Work out the finished part from the listing and answer in its coordinate system (mm). A direction names the side the tool comes from. Coordinates: 2 decimals unless noted, no trailing zeros. Write each loop counter-clockwise with the first axis right and the second up, starting at its lowest first coordinate (ties: lowest second). Pieces come first, ordered by that corner, then holes. Notation, with made-up numbers: (-20, 82) - (2, 82) arc R16 cw to (2, 109) - close; hole circle Ø9 at (37, 62). An arc over 180 degrees is marked (long way). Use one line per item in the form item = value. Start each with the question number.
Item 1: Consider probe 1 along X at (y, z) = (3.25, -6.5); probe 2 along Y at (x, z) = (5.75, -6.25); probe 3 along X at (y, z) = (15.5, -9.25). Determine where each line is inside the solid, lowest interval first.
Item 2: Given pin 1 (2.5 mm diameter, centred on x = 16, z = -8, fed in from +Y); pin 2 (2.5 mm diameter, centred on x = -1.425, z = -7.25, fed in from -Y); pin 3 (5 mm diameter, centred on y = 10.5, z = -1.5, fed in from +X), each flat-ended and moving along its own axis, determine where each tip first touches the part or whether it passes through.
Item 3: A cutting plane is placed at B-B (x = 16.5). Write down the section's boundary in (y, z), then the cut area to 3 significant figures.
Item 4: For faces 5 (the cylindrical face through (8.36, 16.54, -5.02)), 6 (the cylindrical face through (14.398, 7.787, -5.67)), 7 (the flat face through (-3, 0, -7)), 8 (the cylindrical face through (15.31, 1.03, -7.19)), determine the directions among +Z, -Z, +X, -X, +Y, -Y from which every point of the face is accessible in a straight line to the end or side of a thin tool.
Item 5: A cutting plane is placed at D-D (y = 3.5). Write down the section's boundary in (x, z) (3 decimals), then the cut area to 3 significant figures.
Item 6: A cutting plane is placed at A-A (y = -1). Write down the section's boundary in (x, z).
Item 7: A cutting plane is placed at C-C (z = -7.25). Give the number of separate pieces and of enclosed holes in the cut face, then the cut area to 3 significant figures.
Item 8: Determine the mould class of faces 1 (the cylindrical face through (1, 8, -6)), 2 (the cylindrical face through (15.076, 9.547, -7.308)), 3 (the flat face through (7, 12, -11.5)), 4 (the flat face through (7, 11, 0)) for opening direction Z: released by +Z, released by -Z, zero draft, split by the parting line, or undercut.
from build123d import *

# Parameters (mm, degrees)
BOSS_EXTRUDE1_DEPTH      = 11.5
CUT_EXTRUDE1_DEPTH       = 30.162647342
CUT_EXTRUDE1_DEPTH_BACK  = 30.162647342
SKETCH3_R                = 1.05
BOSS_EXTRUDE2_DEPTH      = 3
BOSS_EXTRUDE2_DEPTH_BACK = 11.5
SKETCH4_W                = 3.75
SKETCH4_H                = 3
CUT_EXTRUDE2_DEPTH       = 32.200320548
CUT_EXTRUDE2_DEPTH_BACK  = 32.200320548
SKETCH5_R                = 1.25
CHAMFER1_SIZE            = 6.528307214
CHAMFER1_SIZE_2          = 14
CHAMFER2_SIZE            = 6.528307214
CHAMFER2_SIZE_2          = 14
SKETCH6_R                = 2.6
CUT_EXTRUDE3_DEPTH       = 5
SKETCH7_R                = 1.5
CUT_EXTRUDE4_DEPTH       = 12


with BuildPart() as part:
    # Sketch1 → Boss-Extrude1 (new body)
    with BuildSketch(Plane.XY):
        with BuildLine():
            Line((16.91, 0), (18.9, 0))
            Line((18.9, 0), (18.9, 19))
            Line((18.9, 19), (-3.75, 19))
            Line((-3.75, 19), (-3.75, 0))
            Line((-3.75, 0), (-1.76, 0))
            ThreePointArc((-1.76, 0), (-0.515492065, 0.515492065), (0, 1.76))
            Line((0, 1.76), (0, 6))
            ThreePointArc((0, 6), (0.732233047, 7.767766953), (2.5, 8.5))
            Line((2.5, 8.5), (12.65, 8.5))
            ThreePointArc((12.65, 8.5), (14.417766953, 7.767766953), (15.15, 6))
            Line((15.15, 6), (15.15, 1.76))
            ThreePointArc((15.15, 1.76), (15.665492065, 0.515492065), (16.91, 0))
        make_face()
    extrude(amount=-BOSS_EXTRUDE1_DEPTH)

    # Sketch3 → Cut-Extrude1 (cut, two sides: drawn at the far end of the back side and taken through both)
    with BuildSketch(Plane(origin=(0, 19, 0), x_dir=(1, 0, 0), z_dir=(0, 1, 0)).offset(-CUT_EXTRUDE1_DEPTH_BACK)):
        with Locations(Location((-1.425, 7.25, 0), (0, 0, 251.394661296))):
            Circle(SKETCH3_R)
        with Locations(Location((16.575, 7.25, 0), (0, 0, 288.605338704))):
            Circle(SKETCH3_R)
    extrude(amount=CUT_EXTRUDE1_DEPTH + CUT_EXTRUDE1_DEPTH_BACK, mode=Mode.SUBTRACT)

    # Sketch4 → Boss-Extrude2 (add, two sides: drawn at the far end of the back side and taken through both)
    with BuildSketch(Plane.XZ.offset(-BOSS_EXTRUDE2_DEPTH_BACK)):
        with Locations((17.025, -1.5)):
            Rectangle(SKETCH4_W, SKETCH4_H)
        with Locations((-1.875, -1.5)):
            Rectangle(SKETCH4_W, SKETCH4_H)
    extrude(amount=BOSS_EXTRUDE2_DEPTH + BOSS_EXTRUDE2_DEPTH_BACK)

    # Sketch5 → Cut-Extrude2 (cut, two sides: drawn at the far end of the back side and taken through both)
    with BuildSketch(Plane(origin=(0, 19, 0), x_dir=(1, 0, 0), z_dir=(0, 1, 0)).offset(-CUT_EXTRUDE2_DEPTH_BACK)):
        with Locations(Location((7.575, 7.5, 0), (0, 0, 90))):
            Circle(SKETCH5_R)
    extrude(amount=CUT_EXTRUDE2_DEPTH + CUT_EXTRUDE2_DEPTH_BACK, mode=Mode.SUBTRACT)

    # Chamfer1
    # the kernel refuses this chamfer: 14, 6.528307214 mm, written as the material it takes off along each edge
    with BuildSketch(Plane(origin=(-3.75, 19, 36.2736566), x_dir=(0.9971975577536776, 0.07481330637059945, 0), z_dir=(0, 0, -1))) as chamfer1_piece_1:
        Polygon((CHAMFER1_SIZE * 0.99719755778, CHAMFER1_SIZE * 0.0748133063725), (-CHAMFER1_SIZE_2 * 0.0748133063706, CHAMFER1_SIZE_2 * 0.997197557754), (0, 0), align=None)
    extrude(amount=84.0473132, mode=Mode.SUBTRACT)

    # Chamfer2
    # the kernel refuses this chamfer: 14, 6.528307214 mm, written as the material it takes off along each edge
    with BuildSketch(Plane(origin=(18.9, 19, 36.2736566), x_dir=(-0.9971975577536776, 0.07481330637059945, 0), z_dir=(0, 0, -1))) as chamfer2_piece_1:
        Polygon((CHAMFER2_SIZE * 0.99719755778, -CHAMFER2_SIZE * 0.0748133063725), (-CHAMFER2_SIZE_2 * 0.0748133063706, -CHAMFER2_SIZE_2 * 0.997197557754), (0, 0), align=None)
    extrude(amount=84.0473132, mode=Mode.SUBTRACT)

    # Sketch6 → Cut-Extrude3 (cut)
    with BuildSketch(Plane(origin=(0, 19, 0), x_dir=(1, 0, 0), z_dir=(0, 1, 0))):
        with Locations(Location((7.575, 7.5, 0), (0, 0, 270))):
            Circle(SKETCH6_R)
    extrude(amount=-CUT_EXTRUDE3_DEPTH, mode=Mode.SUBTRACT)

    # Sketch7 → Cut-Extrude4 (cut)
    with BuildSketch(Plane(origin=(0, 19, 0), x_dir=(1, 0, 0), z_dir=(0, 1, 0))):
        with Locations((-1.425, 7.25)):
            Circle(SKETCH7_R)
        with Locations((16.575, 7.25)):
            Circle(SKETCH7_R)
    extrude(amount=-CUT_EXTRUDE4_DEPTH, mode=Mode.SUBTRACT)


solid = part.part
Answer:
q1.probe_1 = -3.75 to -2.16, -0.69 to 0, 15.15 to 15.84, 17.31 to 18.9
q1.probe_2 = 8.5 to 14
q1.probe_3 = 1.15 to 5.65, 9.5 to 14
q2.pin_1 = 13.9
q2.pin_2 = 0
q2.pin_3 = 17.5
q3.outline = (-3, -3) - (0.05, -3) - (0.05, -6.2) - (7, -6.2) - (7, -5.75) - (10.15, -5.75) - (10.15, 0) - (-3, 0) - close; (0.05, -11.5) - (10.15, -11.5) - (10.15, -8.75) - (7, -8.75) - (7, -8.3) - (0.05, -8.3) - close
q3.area = 101 mm²
q4.face_5 = +Y
q4.face_6 = +Z, -Z, -Y
q4.face_7 = -Z, +X, -X, -Y
q4.face_8 = -Z, -Y
q5.outline = (-3.75, -11.5) - (0, -11.5) - (0, 0) - (-3.75, 0) - close; (15.15, -11.5) - (18.9, -11.5) - (18.9, 0) - (15.15, 0) - close; hole circle Ø2.1 at (-1.425, -7.25); hole circle Ø2.1 at (16.575, -7.25)
q5.area = 79.3 mm²
q6.outline = (-3.75, -3) - (0, -3) - (0, 0) - (-3.75, 0) - close; (15.15, -3) - (18.9, -3) - (18.9, 0) - (15.15, 0) - close
q7.separate_pieces = 4
q7.enclosed_holes = 0
q7.area = 125 mm²
q8.face_1 = zero draft
q8.face_2 = undercut
q8.face_3 = released by -Z
q8.face_4 = released by +Z
